Autodesk Inventor part; units mm, degrees
ref_plane "YZ Plane" through (0, 0, 0) normal (1, 0, 0) x (0, 1, 0)
ref_plane "XZ Plane" through (0, 0, 0) normal (0, 1, 0) x (-1, 0, 0)
ref_plane "XY Plane" through (0, 0, 0) normal (0, 0, 1) x (1, 0, 0)
sketch "Sketch1" plane through (0, 0, 0) normal (0, 1, 0) x (-1, 0, 0)
  line L0 (20, 14.965) -> (-20, 14.965)
  line L1 (-20, 14.965) -> (-20, -14.965)
  line L2 (-20, -14.965) -> (20, -14.965)
  line L3 (20, -14.965) -> (20, 14.965)
  point P0 (0, 0)
  dimension "d0" = 29.93
  dimension "d1" = 40
  dimension "d2" = 20
  dimension "d3" = 14.965
extrude "Plate1" add sketch "Sketch1" along normal blind 1.5
sketch "Sketch2" plane through (-20, 0, -13.465) normal (0, 0, -1) x (-1, 0, 0)
  line L0 (-40, 0) -> (0, 0)
  line L1 (0, 0) -> (0, 38.5)
  line L2 (0, 38.5) -> (-40, 38.5)
  line L3 (-40, 38.5) -> (-40, 0)
edge flange "Flange1" height 38.5 angle 90 thickness 1.5 bend radius 0.31 thickness toward (0, 0, -1) relief tear relief width 1.5 relief depth 0.75 corner gap 0.31 corner form 0 edges at (0, 1.5, -14.965) (0, 1.5, 14.965) wall of the first edge with corners at (20, 0, -13.465) (-20, 0, -13.465) (-20, 38.5, -13.465) (20, 38.5, -13.465)
bend "Bend1"
corner "Corner1"
sketch "Sketch3" plane through (-20, 38.5, 14.965) normal (0, 0, 1) x (1, 0, 0)
  line L0 (0, 0) -> (40, 0)
  line L1 (0, -36.69) -> (0, 0)
  circle A0 centre (20, -10) radius 10
  line L2 (0, -28.19) -> (40, -28.19)
  line L3 (40, -28.19) -> (40, -38.19)
  line L4 (40, -38.19) -> (0, -38.19)
  line L5 (0, -38.19) -> (0, -28.19)
  line L6 (40, -28.19) -> (28.9876, -5.6156)
  line L7 (0, -28.19) -> (11.0124, -5.6156)
  line L8 (0, 0) -> (40, 0)
  line L9 (40, 0) -> (40, -35)
  line L10 (40, -35) -> (0, -35)
  line L11 (0, -35) -> (0, 0)
  point P0 (20, -38.5)
  point P1 (20, 0)
  point P2 (0, -28.19)
  point P3 (0, -35)
  point P4 (30, -10)
  dimension "d15" = 10
  dimension "d16" = 0
  dimension "d17" = 20
  dimension "d18" = 18.19
  dimension "d19" = 0
  dimension "d20" = 40
  dimension "d21" = 10
  dimension "d22" = 35
extrude "Extrusion1" cut sketch "Sketch3" against normal blind 35 contours L0 A0 L7 L1 | L0 L9 L6 A0
sketch "Sketch4" plane through (20, 1.81, -14.965) normal (0, 0, -1) x (-1, 0, 0)
  arc A0 (28.9876, 31.0744) -> (11.0124, 31.0744) centre (20, 26.69) ccw
  circle A1 centre (20, 26.69) radius 2.6
  circle A2 centre (13, 26.69) radius 1.05
  circle A3 centre (27, 26.69) radius 1.05
  circle A4 centre (20, 33.69) radius 1.05
  circle A5 centre (20, 19.69) radius 1.05
  point P0 (20, -1.81)
  dimension "d25" = 5.2
  dimension "d26" = 0
  dimension "d27" = 7
  dimension "d28" = 2.1
  dimension "d29" = 7
  dimension "d30" = 0
  dimension "d31" = 2.1
  dimension "d32" = 0
  dimension "d33" = 7
  dimension "d34" = 2.1
  dimension "d35" = 7
  dimension "d36" = 0
  dimension "d37" = 2.1
extrude "Extrusion2" cut sketch "Sketch4" against normal blind 1.5
sketch "Sketch5" plane through (-20, 1.81, 14.965) normal (0, 0, 1) x (1, 0, 0)
  arc A0 (28.9876, 31.0744) -> (11.0124, 31.0744) centre (20, 26.69) ccw
  circle A1 centre (20, 26.69) radius 1.5
  point P0 (20, -1.81)
  dimension "d40" = 3
extrude "Extrusion3" cut sketch "Sketch5" against normal blind 1.5
sketch "Sketch6" plane through (0, 1.5, 0) normal (0, 1, 0) x (1, 0, 0)
  circle A0 centre (-14, -10.155) radius 1.05
  circle A1 centre (-14, -0.75) radius 1.05
  circle A2 centre (-14, 8.655) radius 1.05
  circle A3 centre (14, -10.155) radius 1.05
  circle A4 centre (14, -0.75) radius 1.05
  circle A5 centre (14, 8.655) radius 1.05
  point P0 (0, 0)
hole "Hole1" at (14, 1.5, -8.655) at (14, 1.5, 0.75) at (14, 1.5, 10.155) at (-14, 1.5, 10.155) at (-14, 1.5, 0.75) at (-14, 1.5, -8.655) direction (0, -1, 0) diameter 2.1 depth 1.5
equation "\"d48\" = Thickness"
equation "\"d4\" = Thickness"
equation "\"d5\" = BendReliefWidth"
equation "\"d6\" = BendReliefDepth"
equation "\"d7\" = MinimumRemnant"
equation "\"d8\" = TransitionRadius"
equation "\"d11\" = BendRadius"
equation "\"d12\" = CornerReliefSize"
equation "\"d13\" = GapSize"
equation "\"d14\" = JacobiRadiusSize"
equation "\"BendReliefWidth\" = Thickness"
equation "\"BendReliefDepth\" = 0.5 * Thickness"
equation "\"CornerReliefSize\" = 4 * Thickness"
equation "\"MinimumRemnant\" = 2 * Thickness"
equation "\"TransitionRadius\" = BendRadius"
equation "\"JacobiRadiusSize\" = BendRadius"
equation "\"GapSize\" = Thickness"
properties part number "partpart" material "Aluminum 6061-AHC"
Here's how the part is built. I have some questions about the finished solid (model axes, mm). A direction names the side the tool comes from. Coordinates: 2 decimals unless noted, no trailing zeros. Loops run counter-clockwise (first coordinate to the right, second up) from the corner with the lowest first, then second, coordinate; pieces in that order, holes last.
1. For P1, Ø8, axis at x = -7.5, z = 4, coming from the +Y side; P2, Ø1.3, axis at x = 7, y = 28.5, coming from the -Z side (3 decimals), each with a flat end and sliding along its axis, tell me the tip position at first contact or that it passes through.
2. If we mould it in two halves opening along Z, with no side actions, what happens to faces 4 (the flat face through (-14.57, 21.44, -14.2)), 5 (the flat face through (0, 16, 14.965)), 6 (the cylindrical face through (13.115, 0.74, -8.091)), 7 (the cylindrical face through (-14.89, 0.74, 1.31))? For each: pulls with the +Z half, pulls with the -Z half, needs draft (parallel to the pull), parting line crosses it, or undercut.
3. Imagine slicing it at A-A, the plane z = 10. Please give me the cut outline in (x, y).
4. I need wall thicknesses on L1, parallel to Z at x = -7.5, y = 23.5 (3 decimals); L2, parallel to X at y = 1.1, z = 0.75; L3, parallel to Z at x = -14, y = 0.4 (3 decimals). Which ranges of each line are inside material? Lowest first, please.
5. Imagine slicing it at D-D, the plane y = 28.5. Please give me the cut outline in (x, z) (3 decimals), and give its area (3 significant figures).
6. Imagine slicing it at C-C, the plane x = 7. Please give me the cut outline in (y, z) (3 decimals), and give its area (3 significant figures).
7. For faces 1 (the flat face through (0, 16, -13.465)), 2 (the cylindrical face through (-0.28, 0.544, -14.449)), 3 (the cylindrical face through (7.228, 27.475, -14.226)), which set-ups out of +Z, -Z, +X, -X, +Y, -Y let a thin tool reach every point of the face, with its end or its side?
8. Imagine slicing it at B-B, the plane y = 21.5. Please give me the cut outline in (x, z) (3 decimals).
Taken from the geometry:
1. P1: stops at y = 1.5
1. P2: stops at z = 13.465
2. face 4: needs draft
2. face 5: pulls with the +Z half
2. face 6: undercut
2. face 7: undercut
3. outline: (-20, 0) - (-15.04, 0) - (-15.04, 1.5) - (-20, 1.5) - close; (-12.96, 0) - (12.96, 0) - (12.96, 1.5) - (-12.96, 1.5) - close; (15.04, 0) - (20, 0) - (20, 1.5) - (15.04, 1.5) - close
4. L1: z = -14.965 to -13.465, 13.465 to 14.965
4. L2: x = -20 to -15.05, -12.95 to 12.95, 15.05 to 20
4. L3: z = -14.29 to -9.705, -7.605 to -0.3, 1.8 to 9.105, 11.205 to 14.29
5. outline: (-11.126, -14.965) - (-8.05, -14.965) - (-8.05, -13.465) - (-11.126, -13.465) - close; (-11.126, 13.465) - (-1.5, 13.465) - (-1.5, 14.965) - (-11.126, 14.965) - close; (-5.95, -14.965) - (-2.6, -14.965) - (-2.6, -13.465) - (-5.95, -13.465) - close; (1.5, 13.465) - (11.126, 13.465) - (11.126, 14.965) - (1.5, 14.965) - close; (2.6, -14.965) - (5.95, -14.965) - (5.95, -13.465) - (2.6, -13.465) - close; (8.05, -14.965) - (11.126, -14.965) - (11.126, -13.465) - (8.05, -13.465) - close
5. area: 48.2 mm2
6. outline: (0, -13.155) arc R1.81 ccw to (1.81, -14.965) - (27.45, -14.965) - (27.45, -13.465) - (1.81, -13.465) arc R0.31 cw to (1.5, -13.155) - (1.5, 13.155) arc R0.31 cw to (1.81, 13.465) - (35.641, 13.465) - (35.641, 14.965) - (1.81, 14.965) arc R1.81 ccw to (0, 13.155) - close; (29.55, -14.965) - (35.641, -14.965) - (35.641, -13.465) - (29.55, -13.465) - close
6. area: 143 mm2
7. face 1: +X, -X, +Y
7. face 2: -Z, +X, -X, -Y
7. face 3: -Z
8. outline: (-14.541, -14.965) - (-1.05, -14.965) - (-1.05, -13.465) - (-14.541, -13.465) - close; (-14.541, 13.465) - (14.541, 13.465) - (14.541, 14.965) - (-14.541, 14.965) - close; (1.05, -14.965) - (14.541, -14.965) - (14.541, -13.465) - (1.05, -13.465) - close
